Can you work these out from the drawing? Everything is in mm from the part's minimum corner. A direction names the side the tool comes from. Coordinates: 2 decimals unless noted, no trailing zeros. Loops run counter-clockwise (first coordinate to the right, second up) from the corner with the lowest first, then second, coordinate; pieces in that order, holes last.
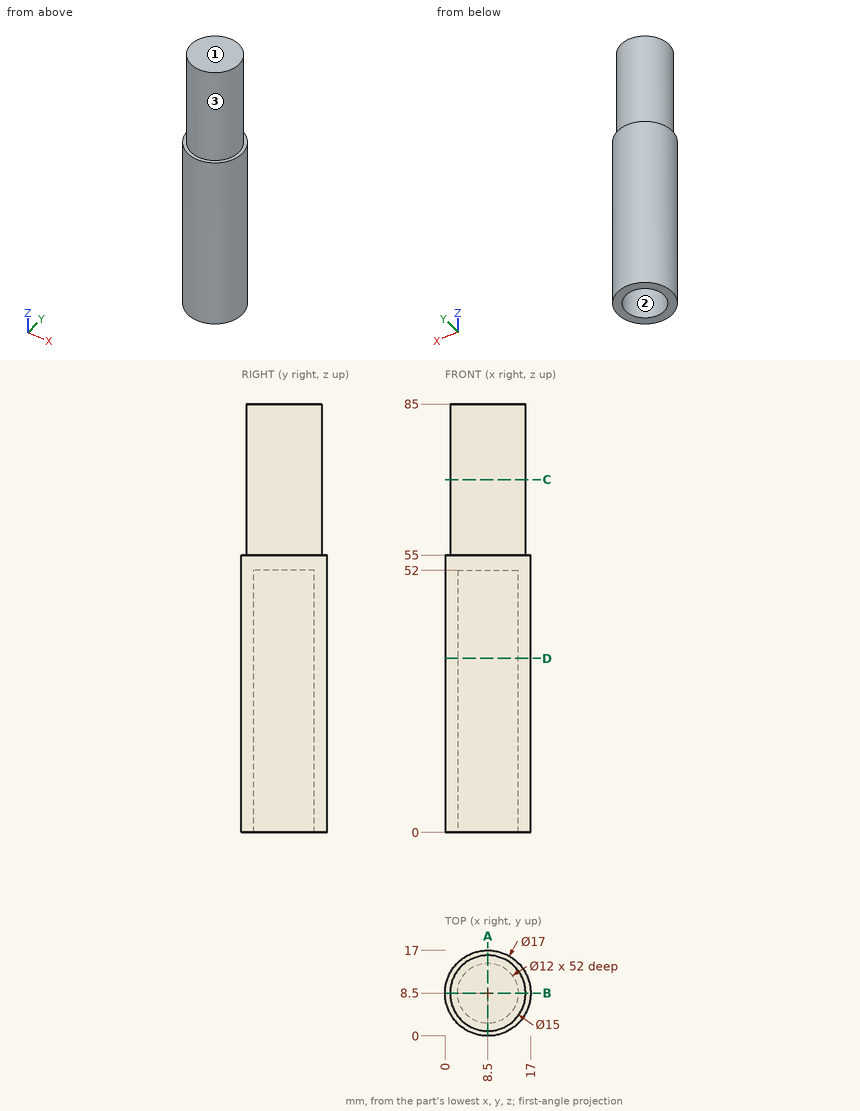
(1) Which directions (+Z, -Z, +X, -X, +Y, -Y) give clear straight access to the entire face, cutting with the end or side of a thin tool? Please do the marked faces 1, 2 and 3.
Answers:
face 1: +Z, +X, -X, +Y, -Y
face 2: -Z
face 3: +Z
(2) I need wall thicknesses on probe 1 along Z at (x, y) = (11.75, 8.5); probe 2 along Y at (x, z) = (8.5, 28.5); probe 3 along Z at (x, y) = (13.25, 15.25). Which ranges of each line are inside material? Lowest first, please.
Answers:
probe 1: z = 52 to 85
probe 2: y = 0 to 2.5, 14.5 to 17
probe 3: z = 0 to 55
(3) Imagine slicing it at D-D, the plane z = 34.5. Write out the boundary of the cut face in (x, y).
Answers:
outline: circle Ø17 at (8.5, 8.5); hole circle Ø12 at (8.5, 8.5)
(4) For pin 1 (1.5 mm diameter, centred on x = 12.5, z = 32.5, fed in from -Y); pin 2 (5 mm diameter, centred on y = 5, z = 10.5, fed in from +X); pin 3 (2 mm diameter, centred on y = 5.5, z = 66.5, fed in from -X); pin 4 (4 mm diameter, centred on y = 10.5, z = 11.5, fed in from -X), each with a flat end and sliding along its axis, tell me the tip position at first contact or that it passes through.
Answers:
pin 1: stops at y = 0.65
pin 2: stops at x = 16.94
pin 3: stops at x = 1.27
pin 4: stops at x = 0
(5) Imagine slicing it at C-C, the plane z = 70. Write out the boundary of the cut face in (x, y).
Answers:
outline: circle Ø15 at (8.5, 8.5)
(6) Imagine slicing it at A-A, the plane x = 8.5. Write out the boundary of the cut face in (y, z).
Answers:
outline: (0, 0) - (2.5, 0) - (2.5, 52) - (14.5, 52) - (14.5, 0) - (17, 0) - (17, 55) - (16, 55) - (16, 85) - (1, 85) - (1, 55) - (0, 55) - close
